from build123d import *

# Parameters (mm, degrees)
F0_R     = 72
F1_DEPTH = 40
F2_R     = 78
F3_DEPTH = 10


with BuildPart() as f1:
    # F0 (on Top) → F1 (new body)
    with BuildSketch(Plane.XY):
        Circle(F0_R)
    extrude(amount=F1_DEPTH)

    # F2 (on face) → F3 (join)
    with BuildSketch(Plane.XY.offset(40)):
        Circle(F2_R)
    extrude(amount=F3_DEPTH)

    # F4 (on Front) → F5 (revolve, cut)
    with BuildSketch(Plane.XZ):
        Polygon((70.5, 50), (0, 50), (0, 0), (62.5, 0), (62.5, 42), align=None)
    revolve(axis=Axis((0, 0, 50), (0, 0, 1)), mode=Mode.SUBTRACT)


solid = f1.part
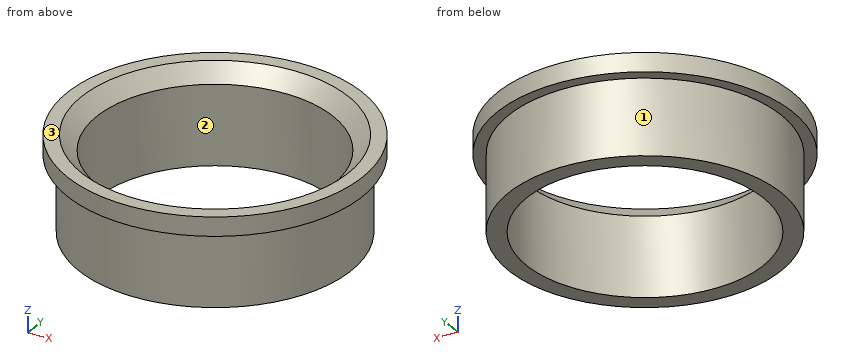
Part model, mm, in its own coordinate system. Face numbers are marked on the shaded views. Coordinates: 2 decimals unless noted, no trailing zeros. Order: outer loops, then holes, each group sorted by start corner. A loop starts at its lowest first (then second) coordinate and runs counter-clockwise, first axis right, second up.
(1) Slice it at A-A, the plane y = 0. Write the cut outline in (x, z), and give its area (3 significant figures).
Check sheet entries:
outline: (-78, 40) - (-72, 40) - (-72, 0) - (-62.5, 0) - (-62.5, 42) - (-70.5, 50) - (-78, 50) - close; (62.5, 0) - (72, 0) - (72, 40) - (78, 40) - (78, 50) - (70.5, 50) - (62.5, 42) - close
area: 1,010 mm2
(2) Probe L1, parallel to Y at x = 0, z = 33; L2, parallel to Y at x = -10, z = 41.5; L3, parallel to X at y = 4.5, z = 7.5. List the from-to ranges inside material, lowest first.
Check sheet entries:
L1: y = -72 to -62.5, 62.5 to 72
L2: y = -77.36 to -61.69, 61.69 to 77.36
L3: x = -71.86 to -62.34, 62.34 to 71.86
(3) Pin check, flat tips, straight feed: pin 1 Ø1.5 at (y, z) = (-34.5, 10) entering from +X; pin 2 Ø12 at (x, z) = (10, 13) entering from -Y; pin 3 Ø10 at (y, z) = (-57.5, 42) entering from +X. Stop position of each tip, or through.
Check sheet entries:
pin 1: stops at x = 63.6
pin 2: stops at y = -71.89
pin 3: stops at x = 57.69
(4) Pull direction Y, two halves, no side cores. Call the marked faces 1, 2 and 3: pulls with the +Y half, pulls with the -Y half, needs draft (parallel to the pull), parting line crosses it, or undercut.
Check sheet entries:
face 1: parting line crosses it
face 2: undercut
face 3: needs draft
(5) Slice it at D-D, the plane z = 46. Write the cut outline in (x, y).
Check sheet entries:
outline: circle Ø156 at (0, 0); hole circle Ø133 at (0, 0)
(6) Slice it at C-C, the plane z = 17. Write the cut outline in (x, y).
Check sheet entries:
outline: circle Ø144 at (0, 0); hole circle Ø125 at (0, 0)
